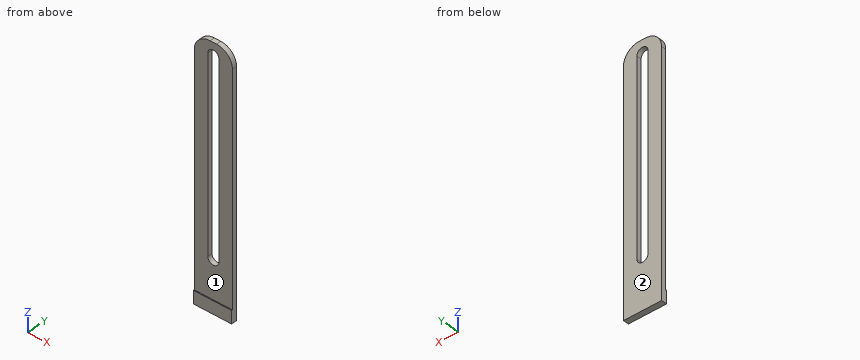
from build123d import *

# Parameters (mm, degrees)
EXTRUDE_1_DEPTH = 1.5
SKETCH_2_W      = 12
SKETCH_2_H      = 4
EXTRUDE_2_DEPTH = 0.3


with BuildPart() as part:
    # 草图1 → 凸台-拉伸1 (new body)
    with BuildSketch(Plane(origin=(0, 0, 0), x_dir=(1, 0, 0), z_dir=(0, 1, 0))):
        with BuildLine():
            Line((-6, 40), (6, 40))
            Line((6, 40), (6, -35))
            ThreePointArc((6, -35), (4.535533906, -38.535533906), (1, -40))
            Line((1, -40), (-1, -40))
            ThreePointArc((-1, -40), (-4.535533906, -38.535533906), (-6, -35))
            Line((-6, -35), (-6, 40))
        make_face()
        with BuildLine():
            Line((-1.75, -36), (-1.75, 24))
            ThreePointArc((-1.75, 24), (0, 25.75), (1.75, 24))
            Line((1.75, 24), (1.75, -36))
            ThreePointArc((1.75, -36), (0, -37.75), (-1.75, -36))
        make_face(mode=Mode.SUBTRACT)
    extrude(amount=EXTRUDE_1_DEPTH)

    # 草图2 → 凸台-拉伸2 (add)
    with BuildSketch(Plane.XZ):
        with Locations((0, -38)):
            Rectangle(SKETCH_2_W, SKETCH_2_H)
    extrude(amount=EXTRUDE_2_DEPTH)


solid = part.part
Work out the finished part from the listing and answer in its coordinate system (mm). Face numbers are marked on the shaded views. A direction names the side the tool comes from. Round coordinates to 2 decimals unless told otherwise and drop trailing zeros. Order: outer loops, then holes, each group sorted by start corner. A loop starts at its lowest first (then second) coordinate and runs counter-clockwise, first axis right, second up. Notation, with made-up numbers: M 60.25,19.5 L 90.25,19.5 A5 cw 90.25,27.5 Z; hole C -38,32 d2. An arc over 180 degrees is marked long. Put each result on its own line as item: value. Start each with the question number.
Q1. A tool of negligible diameter and unlimited length cuts with its end or side. For the marked faces 1 and 2, from which of +Z, -Z, +X, -X, +Y, -Y can it reach the whole face along a straight path? Write none if from no direction.
Q2. Section C-C, the plane y = 0.7 is taken. Write down the section's boundary in (x, z).
Q3. Straight lines are drawn through the part: L1, parallel to X at y = 1.4, z = 13.5; L2, parallel to Y at x = 5, z = 31; L3, parallel to Z at x = -1, y = 0.65. For each, find the intervals that lie inside material, in ascending order. Write a range as [from, to].
Q4. A flat-ended cylindrical pin translates along its axis: pin 1 (6 mm diameter, centred on x = 1, z = -6.5, fed in from -Y). Find the tip coordinate at first contact, or state that the pin passes through.
Q5. Section B-B, the plane z = 18 is taken. Write down the section's boundary in (x, y).
Q6. Section A-A, the plane x = 0 is taken. Write down the section's boundary in (y, z), and give its area (4 significant figures).
Findings below:
1. face 1: +Z, +X, -X, -Y
1. face 2: +Z, -Z, +X, -X, +Y
2. outline: M -6,-40 L 6,-40 L 6,35 A5 ccw 1,40 L -1,40 A5 ccw -6,35 Z; hole M -1.75,-24 A1.75 ccw 1.75,-24 L 1.75,36 A1.75 ccw -1.75,36 Z
3. L1: x = [-6, -1.75], [1.75, 6]
3. L2: y = [0, 1.5]
3. L3: z = [-40, -25.44], [37.44, 40]
4. pin 1: stops at y = 0
5. outline: M -6,0 L -1.75,0 L -1.75,1.5 L -6,1.5 Z; M 1.75,0 L 6,0 L 6,1.5 L 1.75,1.5 Z
6. outline: M -0.3,-40 L 1.5,-40 L 1.5,-25.75 L 0,-25.75 L 0,-36 L -0.3,-36 Z; M 0,37.75 L 1.5,37.75 L 1.5,40 L 0,40 Z
6. area: 25.95 mm^2
